```python
from build123d import *

# Parameters (mm, degrees)
F4_W          = 1.2
F4_H          = 19.620869044
F5_DEPTH      = 25
F5_DEPTH_BACK = 25


# Not quite as in the source:
# - a fillet or chamfer that OpenCascade refuses, or shapes differently, is made with other operations: its cross-section is extruded or revolved along the edge and cut away or added


with BuildPart() as f2:
    # F2: sweep along a path in F0
    with BuildLine(Plane.XZ) as f2_path:
        CenterArc((0, 0), 8.875, 0, 360)
    # F1 (on Right) → F2 (sweep)
    with BuildSketch(Plane.YZ):
        Polygon((-2.5, 8.4675319269), (0, 8.4675319269), (2.5, 8.4675319269), (2.7924242295, 10.246030055), (0.65, 10.7327634469), (0.65, 9.5877971399), (0.494154765, 9.4675319269), (0, 9.4675319269), (-0.494154765, 9.4675319269), (-0.65, 9.5877971399), (-0.65, 10.7327634469), (-2.7924242295, 10.246030055), align=None)
    sweep(path=f2_path.line)

    # F3: fillet of radius 2.0708896165 on 2 edges, made by hand

    # F3_s1 → F3_t2 (revolve, cut)
    with BuildSketch(Plane.XY):
        with BuildLine():
            ThreePointArc((10.6767355553, -0.8966145009), (9.8737027886, -2.1138201975), (8.4675319269, -2.5))
            Line((8.4675319269, -2.5), (10.246030055, -2.7924242295))
            Line((10.246030055, -2.7924242295), (10.6767355553, -0.8966145009))
        make_face()
    revolve(axis=Axis((0, -2.7924242295, 0), (0, -1, 0)), mode=Mode.SUBTRACT)

    # F3_s3 → F3_t4 (revolve, cut)
    with BuildSketch(Plane.XY):
        with BuildLine():
            ThreePointArc((8.4675319269, 2.5), (9.8737027886, 2.1138201975), (10.6767355553, 0.8966145009))
            Line((10.6767355553, 0.8966145009), (10.246030055, 2.7924242295))
            Line((10.246030055, 2.7924242295), (8.4675319269, 2.5))
        make_face()
    revolve(axis=Axis((0, 2.7924242295, 0), (0, -1, 0)), mode=Mode.SUBTRACT)

    # F4 (on Front) → F5 (cut, two sides)
    with BuildSketch(Plane.XZ) as f5_sk:
        Rectangle(F4_W, F4_H)
    extrude(amount=-F5_DEPTH, mode=Mode.SUBTRACT)
    extrude(f5_sk.sketch, amount=F5_DEPTH_BACK, mode=Mode.SUBTRACT)


solid = f2.part
```
Verification items for the finished model (mm, model axes). A direction names the side the tool comes from. Coordinates: 2 decimals unless noted, no trailing zeros. Order: outer loops, then holes, each group sorted by start corner. A loop starts at its lowest first (then second) coordinate and runs counter-clockwise, first axis right, second up. Notation, with made-up numbers: (55, 22) -> (82, 22) arc R21 cw to (82, 59) -> close; hole circle Ø8 at (-18.75, 47). An arc over 180 degrees is marked (long way). Put each result on its own line as item: value. Start each with the question number.
1) Cross-section at A-A (y = 0.2). Enter the section's corners in (x, z), plus the area to 3 significant figures.
2) Release check for a two-part mould opening along Y. For faces 3 (the flat face through (-0.6, 0, -9)), 4 (the cylindrical face through (-9.465, -0.007, 0.2)) record: pulls with the +Y half, pulls with the -Y half, needs draft (parallel to the pull), parting line crosses it, or undercut.
3) Cross-section at B-B (x = 0). State how many separate pieces and enclosed holes the cut face has, plus the area to 3 significant figures.
4) Material ranges on L1, parallel to X at y = -1.8, z = -2.75; L2, parallel to X at y = 1.85, z = -0.75; L3, parallel to Z at x = -3.5, y = 0.85, recorded low to high.
5) Tool access check on faces 1 (the flat face through (0, 1, 9.81)), 2 (the cylindrical face through (9.465, -0.007, -0.2)). Record the directions out of +Z, -Z, +X, -X, +Y, -Y that give a thin tool (end or side, any length) a straight path to the whole face; none if there is none.
6) Go/stop test with flat-tipped pins: pin 1 (0.7 mm diameter, centred on y = 1, z = -9.5, fed in from -X); pin 2 (0.6 mm diameter, centred on x = 0, y = -1.5, fed in from +Z); pin 3 (1 mm diameter, centred on x = 5, y = -1, fed in from -Z). Record where each tip stops, or that it passes through.
Geometry check:
1. outline: (-0.6, -9.45) -> (-0.6, -8.45) arc R8.47 cw to (-0.6, 8.45) -> (-0.6, 9.45) arc R9.47 ccw to start; (0.6, -9.45) arc R9.47 ccw to (0.6, 9.45) -> (0.6, 8.45) arc R8.47 cw to (0.6, -8.45) -> close
1. area: 53.9 mm^2
2. face 3: needs draft
2. face 4: undercut
3. separate pieces: 4
3. enclosed holes: 0
3. area: 3.67 mm^2
4. L1: x = -9.84 to -8.01, 8.01 to 9.84
4. L2: x = -10.14 to -8.43, 8.43 to 10.14
4. L3: z = -10.1 to -7.71, 7.71 to 10.1
5. face 1: +Y, -Y
5. face 2: +X
6. pin 1: stops at x = -5.48
6. pin 2: stops at z = 10.58
6. pin 3: stops at z = -9.69
